```python
from build123d import *

# Parameters (mm, degrees)
CHAMFER1_SIZE = 0.5


with BuildPart() as part:
    # Sketch1 → Revolve1 (revolve)
    with BuildSketch(Plane.XY):
        with BuildLine():
            Line((-2.5, 11), (-2.190319611, 11))
            ThreePointArc((-2.190319611, 11), (0, 10.05), (2.190319611, 11))
            Line((2.190319611, 11), (2.5, 11))
            Line((2.5, 11), (2.5, 7))
            Line((2.5, 7), (-2.5, 7))
            Line((-2.5, 7), (-2.5, 11))
        make_face()
    revolve(axis=Axis((-15.9375, 0, 0), (1, 0, 0)))

    # Chamfer1
    chamfer1_edges = [part.edges().sort_by_distance(p)[0] for p in [
        (2.5, -7, 0),
        (-2.5, -7, 0),
    ]]
    chamfer(chamfer1_edges, length=CHAMFER1_SIZE)


solid = part.part
```
The listing builds one solid part. Answer for the finished solid, in the listing's coordinates (mm). Round coordinates to 2 decimals unless told otherwise and drop trailing zeros. Loops run counter-clockwise (first coordinate to the right, second up) from the corner with the lowest first, then second, coordinate; pieces in that order, holes last. Notation, with made-up numbers: (19, -26) - (71, -26) arc R19 ccw to (71, 8) - close; hole circle Ø5 at (49, 33). An arc over 180 degrees is marked (long way). Return JSON: item names as keys, results as strings. Group by question number.
1. The part is cut by section D-D on x = -1.25. Determine the outline of the cut face in (y, z), then the cut area to 3 significant figures.
2. Consider probe 1 along Y at (x, z) = (-0.9, 2.5); probe 2 along Y at (x, z) = (-1, -1.5); probe 3 along Z at (x, y) = (-0.25, 0). Determine where each line is inside the solid, lowest interval first.
3. The part is cut by section A-A on z = 0. Determine the outline of the cut face in (x, y), then the cut area to 3 significant figures.
4. Each of these flat-tipped pins is pushed along its axis until it touches: P1, Ø1.5, axis at x = 0, y = 8, coming from the -Z side; P2, Ø1, axis at x = -1, z = 1.5, coming from the -Y side. Where does it stop, or does it pass through?
5. The part is cut by section C-C on x = 0.2. Determine the outline of the cut face in (y, z), then the cut area to 3 significant figures.
6. The mould has two halves that part along Y. Classify faces 1 (the cylindrical face through (-2.343, -2.385, -10.738)), 2 (the flat face through (-2.5, -7.2, 2.6)), 3 (the cylindrical face through (-0.028, 6.466, -2.681)): pulls with the +Y half, pulls with the -Y half, needs draft (parallel to the pull), parting line crosses it, or undercut.
Resolved:
{
 "1": {"outline": "circle Ø20.65 at (0, 0); hole circle Ø14 at (0, 0)", "area": "181 mm²"},
 "2": {"probe 1": "y = -9.88 to -6.54, 6.54 to 9.88", "probe 2": "y = -10.11 to -6.84, 6.84 to 10.11", "probe 3": "z = -10.06 to -7, 7 to 10.06"},
 "3": {"outline": "(-2.5, -11) - (-2.19, -11) arc R3 cw to (2.19, -11) - (2.5, -11) - (2.5, -7.5) - (2, -7) - (-2, -7) - (-2.5, -7.5) - close; (-2.5, 7.5) - (-2, 7) - (2, 7) - (2.5, 7.5) - (2.5, 11) - (2.19, 11) arc R3 cw to (-2.19, 11) - (-2.5, 11) - close", "area": "33.7 mm²"},
 "4": {"P1": "stops at z = -6.96", "P2": "stops at y = -10.35"},
 "5": {"outline": "circle Ø20.11 at (0, 0); hole circle Ø14 at (0, 0)", "area": "164 mm²"},
 "6": {"face 1": "parting line crosses it", "face 2": "needs draft", "face 3": "undercut"}
}
